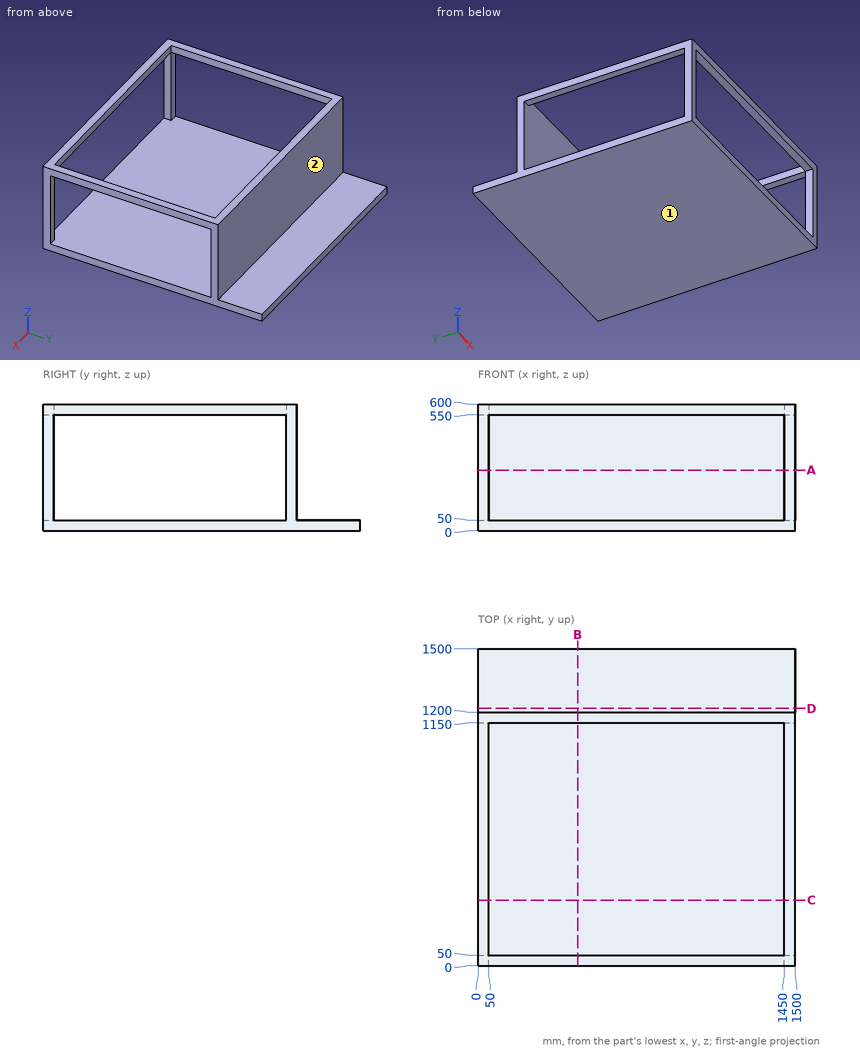
Input: dimensioned drawing with shaded views. Units: mm. Origin: part minimum x, y, z. A direction names the side the tool comes from. Round coordinates to 2 decimals unless told otherwise and drop trailing zeros. Loops run counter-clockwise (first coordinate to the right, second up) from the corner with the lowest first, then second, coordinate; pieces in that order, holes last. Notation, with made-up numbers: M 80,68 L 98,68 A12 cw 98,81 Z; hole C -31.75,-31.5 d3. An arc over 180 degrees is marked long. Return JSON: item names as keys, results as strings. Group by question number.
1. Section query D-D on y = 1218.5. Output: boundary loops of the cut face in (x, z), and give its area (3 significant figures).
2. Section query A-A on z = 287.5. Output: boundary loops of the cut face in (x, y), and give its area (3 significant figures).
3. Reachability of the marked faces 1 and 2 from +Z, -Z, +X, -X, +Y, -Y: full face, straight path, thin tool, end or side. Return the list, or none.
4. Pin query (flat end, axial travel): pin 1 (2 mm diameter, centred on x = 1189.5, z = 525.5, fed in from +Y); pin 2 (5 mm diameter, centred on x = 1302.5, z = 374, fed in from -Y). Return the tip coordinate at first contact, or that it passes through.
5. Section query B-B on x = 471.5. Output: boundary loops of the cut face in (y, z), and give its area (3 significant figures).
6. Section query C-C on y = 311. Output: boundary loops of the cut face in (x, z).
7. Material intervals for line 1 along X through (y, z) = (494.5, 560.5); line 2 along Y through (x, z) = (1122, 529); line 3 along Z through (x, y) = (1216.5, 537.5), sorted ascending. Write a range as from..to.
Checks:
{
 "1": {"outline": "M 0,0 L 1500,0 L 1500,50 L 0,50 Z", "area": "75,000 mm²"},
 "2": {"outline": "M 0,0 L 50,0 L 50,50 L 0,50 Z; M 0,1150 L 1500,1150 L 1500,1200 L 0,1200 Z; M 1450,0 L 1500,0 L 1500,50 L 1450,50 Z", "area": "80,000 mm²"},
 "3": {"face 1": "-Z, +X, -X, +Y, -Y", "face 2": "+Z, +X, -X, +Y"},
 "4": {"pin 1": "stops at y = 1200", "pin 2": "stops at y = 1150"},
 "5": {"outline": "M 0,0 L 1500,0 L 1500,50 L 1200,50 L 1200,600 L 1150,600 L 1150,50 L 0,50 Z; M 0,550 L 50,550 L 50,600 L 0,600 Z", "area": "105,000 mm²"},
 "6": {"outline": "M 0,0 L 1500,0 L 1500,50 L 0,50 Z; M 0,550 L 50,550 L 50,600 L 0,600 Z; M 1450,550 L 1500,550 L 1500,600 L 1450,600 Z"},
 "7": {"line 1": "x = 0..50, 1450..1500", "line 2": "y = 1150..1200", "line 3": "z = 0..50"}
}
